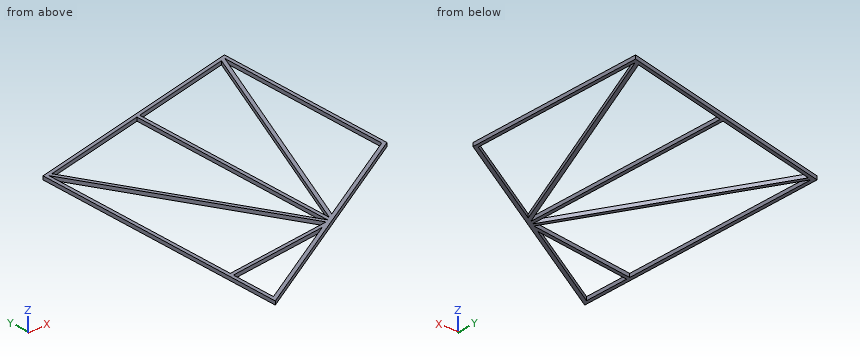
from build123d import *

# Parameters (mm, degrees)
EXTRUDE_1_DEPTH = 2


with BuildPart() as part:
    # ｽｹｯﾁ1 → ﾎﾞｽ - 押し出し1 (new body)
    with BuildSketch(Plane.XY):
        Polygon((130, 75.055534995), (0, 0), (0, 150), (130, 180.012864846), align=None)
        Polygon((128, 76.210235533), (2, 3.464101615), (2, 148.409128167), (128, 177.498520248), align=None, mode=Mode.SUBTRACT)
        Polygon((67, 163.41556059), (65, 162.953824208), (65, 39.837168574), (67, 40.991869112), align=None)
        Polygon((4.029439999, 148.877661308), (2, 148.409128167), (63.267785356, 38.837073983), (65, 39.837168574), align=None)
        Polygon((125.581629022, 176.940195315), (67, 40.991869112), (69.899019864, 42.665619011), (128, 177.498520248), align=None)
        Polygon((63.267785356, 38.837073983), (2, 31.314335861), (2, 29.29931621), (58.834939644, 36.277769318), align=None)
    extrude(amount=EXTRUDE_1_DEPTH)


solid = part.part
The listing builds one solid part. Answer for the finished solid, in the listing's coordinates (mm). Round coordinates to 2 decimals unless told otherwise and drop trailing zeros. Order: outer loops, then holes, each group sorted by start corner. A loop starts at its lowest first (then second) coordinate and runs counter-clockwise, first axis right, second up. Notation, with made-up numbers: (32, -38) - (81, -38) arc R38 ccw to (81, 0) - close; hole circle Ø9 at (37, 44). An arc over 180 degrees is marked (long way). Write item = value, one per line. Start each with the question number.
1) Straight lines are drawn through the part: L1, parallel to Y at x = 33.5, z = 0.45; L2, parallel to X at y = 132.5, z = 0.8; L3, parallel to Y at x = 56, z = 1.2. For each, find the intervals that lie inside material, in ascending order.
2) Section D-D, the plane x = 52 is taken. Write down the section's boundary in (y, z), plus the area to 3 significant figures.
3) Section C-C, the plane z = 0.4 is taken. Write down the section's boundary in (x, y), plus the area to 3 significant figures.
4) Section B-B, the plane y = 118 is taken. Write down the section's boundary in (x, z), plus the area to 3 significant figures.
5) Section A-A, the plane x = 72 is taken. Write down the section's boundary in (y, z), plus the area to 3 significant figures.
Results list:
q1.L1 = 19.34 to 21.65, 33.17 to 35.18, 92.07 to 96.17, 155.68 to 157.73
q1.L2 = 0 to 2, 10.9 to 13.19, 65 to 67, 106.43 to 108.61, 128 to 130
q1.L3 = 32.33 to 34.64, 35.93 to 37.94, 51.83 to 55.93, 160.88 to 162.93
q2.outline = (30.02, 0) - (32.33, 0) - (32.33, 2) - (30.02, 2) - close; (35.44, 0) - (37.45, 0) - (37.45, 2) - (35.44, 2) - close; (58.99, 0) - (63.09, 0) - (63.09, 2) - (58.99, 2) - close; (159.95, 0) - (162.01, 0) - (162.01, 2) - (159.95, 2) - close
q2.area = 21.0 mm^2
q3.outline = (0, 0) - (130, 75.06) - (130, 180.01) - (0, 150) - close; hole (2, 3.46) - (58.83, 36.28) - (2, 29.3) - close; hole (2, 31.31) - (63.27, 38.84) - (2, 148.41) - close; hole (4.03, 148.88) - (65, 39.84) - (65, 162.95) - close; hole (67, 40.99) - (125.58, 176.94) - (67, 163.42) - close; hole (69.9, 42.67) - (128, 76.21) - (128, 177.5) - close
q3.area = 1,970 mm^2
q4.outline = (0, 0) - (2, 0) - (2, 2) - (0, 2) - close; (19, 0) - (21.29, 0) - (21.29, 2) - (19, 2) - close; (65, 0) - (67, 0) - (67, 2) - (65, 2) - close; (100.18, 0) - (102.36, 0) - (102.36, 2) - (100.18, 2) - close; (128, 0) - (130, 0) - (130, 2) - (128, 2) - close
q4.area = 20.9 mm^2
q5.outline = (41.57, 0) - (43.88, 0) - (43.88, 2) - (41.57, 2) - close; (47.54, 0) - (52.6, 0) - (52.6, 2) - (47.54, 2) - close; (164.57, 0) - (166.62, 0) - (166.62, 2) - (164.57, 2) - close
q5.area = 18.8 mm^2
